Part model, mm, in its own coordinate system. Face numbers are marked on the shaded views. A direction names the side the tool comes from. Round coordinates to 2 decimals unless told otherwise and drop trailing zeros. Order: outer loops, then holes, each group sorted by start corner. A loop starts at its lowest first (then second) coordinate and runs counter-clockwise, first axis right, second up. Notation, with made-up numbers: (-1.5, -37) - (40.5, -37) arc R17 ccw to (40.5, -20) - close; hole circle Ø6 at (61, 36.5). An arc over 180 degrees is marked (long way). Answer as a JSON object with one key per item and string values.
```python
from build123d import *

# Parameters (mm, degrees)
F0_R     = 13.25
F1_DEPTH = 10
F2_W     = 6.9995252416
F2_H     = 11.4660244435
F3_DEPTH = 5
F4_R     = 1.115966898
F5_DEPTH = 7.5
F6_R     = 2
F7_R     = 1


with BuildPart() as f1:
    # F0 (on Top) → F1 (new body)
    with BuildSketch(Plane.XY):
        Circle(F0_R)
    extrude(amount=F1_DEPTH)

    # F2 (on face) → F3 (join)
    with BuildSketch(Plane(origin=(0, 0, 0), x_dir=(1, 0, 0), z_dir=(0, 0, -1))):
        Rectangle(F2_W, F2_H)
    extrude(amount=F3_DEPTH)

    # F4 (on Right) → F5 (join, symmetric)
    with BuildSketch(Plane.YZ):
        with Locations((0, -2.5976826437)):
            Circle(F4_R)
    extrude(amount=F5_DEPTH, both=True)

    # F6
    f6_edges = [f1.edges().sort_by_distance(p)[0] for p in [
        (-13.25, 0, 0),
    ]]
    fillet(f6_edges, radius=F6_R)

    # F7
    f7_edges = [f1.edges().sort_by_distance(p)[0] for p in [
        (0, 5.733012, -5),
        (3.499763, 0, -5),
        (0, -5.733012, -5),
        (-3.499763, 0, -5),
    ]]
    fillet(f7_edges, radius=F7_R)


solid = f1.part
```
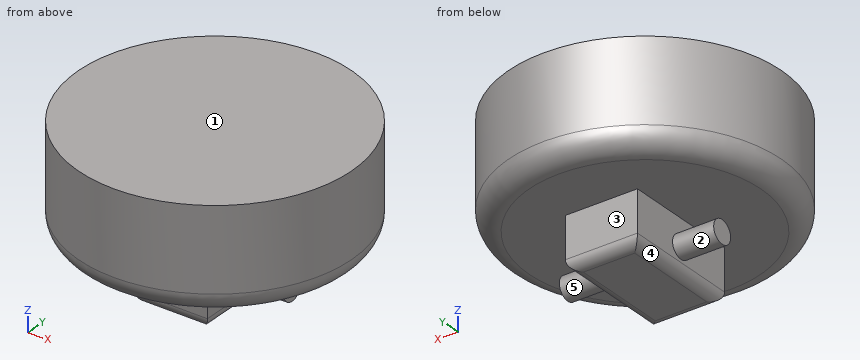
Item 1: Tool access for the marked faces 1 and 2: list every direction of +Z, -Z, +X, -X, +Y, -Y with a clear straight run to the whole face (end or side of a thin tool).
Taken from the geometry:
{"face 1": "+Z, +X, -X, +Y, -Y", "face 2": "-X"}
Item 2: Cut at B-B (y = 0). Write the cut outline in (x, z), plus the area to 3 significant figures.
Taken from the geometry:
{"outline": "(-13.25, 2) arc R2 ccw to (-11.25, 0) - (-3.5, 0) - (-3.5, -1.48) - (-7.5, -1.48) - (-7.5, -3.71) - (-3.5, -3.71) - (-3.5, -4) arc R1 ccw to (-2.5, -5) - (2.5, -5) arc R1 ccw to (3.5, -4) - (3.5, -3.71) - (7.5, -3.71) - (7.5, -1.48) - (3.5, -1.48) - (3.5, 0) - (11.25, 0) arc R2 ccw to (13.25, 2) - (13.25, 10) - (-13.25, 10) - close", "area": "316 mm2"}
Item 3: Cut at A-A (x = 0). Write the cut outline in (y, z).
Taken from the geometry:
{"outline": "(-13.25, 2) arc R2 ccw to (-11.25, 0) - (-5.73, 0) - (-5.73, -4) arc R1 ccw to (-4.73, -5) - (4.73, -5) arc R1 ccw to (5.73, -4) - (5.73, 0) - (11.25, 0) arc R2 ccw to (13.25, 2) - (13.25, 10) - (-13.25, 10) - close"}
Item 4: Probe L1, parallel to Z at x = 6, y = 6.25; L2, parallel to X at y = -0.25, z = -0.75; L3, parallel to X at y = -6.75, z = 1.25. List the from-to ranges inside material, lowest first. Write a range as from..to.
Taken from the geometry:
{"L1": "0..10", "L2": "-3.5..3.5", "L3": "-11.23..11.23"}
Item 5: Two-plate mould, pull along Z, no slides. Class the marked faces 3, 4 and 5: pulls with the +Z half, pulls with the -Z half, needs draft (parallel to the pull), parting line crosses it, or undercut.
Taken from the geometry:
{"face 3": "needs draft", "face 4": "pulls with the -Z half", "face 5": "undercut"}
Item 6: Drop flat-ended pins along their axis: P1, Ø4.5, axis at y = 1, z = -2, coming from the -X side; P2, Ø1.5, axis at x = -7, z = -1.5, coming from the +Y side; P3, Ø3, axis at x = -0.5, z = -1, coming from the -Y side; P4, Ø8, axis at y = 2, z = 6.5, coming from the -X side. Give the stop position or say it passes through.
Taken from the geometry:
{"P1": "x = -12.18", "P2": "y = 1.06", "P3": "y = -12.56", "P4": "x = -13.25"}
Item 7: Cut at C-C (z = 8.5). Write the cut outline in (x, y).
Taken from the geometry:
{"outline": "circle Ø26.5 at (0, 0)"}
